Can you work these out from the model? Positions are in its coordinate system, mm. Face numbers are marked on the shaded views. A direction names the side the tool comes from. Round coordinates to 2 decimals unless told otherwise and drop trailing zeros. Write each loop counter-clockwise with the first axis right and the second up, starting at its lowest first coordinate (ties: lowest second). Pieces come first, ordered by that corner, then holes. Notation, with made-up numbers: M 14,-3 L 45,-3 A21 cw 45,13 Z; hole C 10.25,-27.5 d3. An arc over 180 degrees is marked long. Answer in a Markdown table with one row per item. Add a question column.
(1) Suppose I cut it at D-D, the plane z = 15. Write out the boundary of the cut face in (x, y).
(2) Suppose I cut it at A-A, the plane y = 0. Write out the boundary of the cut face in (x, z), then the cut area to 3 significant figures.
(3) Suppose I cut it at C-C, the plane z = 5. Write out the boundary of the cut face in (x, y), then the cut area to 3 significant figures.
(4) For the marked faces 1, 2 and 3, which set-ups out of +Z, -Z, +X, -X, +Y, -Y let a thin tool reach every point of the face, with its end or its side?
(5) If I drill on probe 1 along Y at (x, z) = (0, 7); probe 2 along Z at (x, y) = (-38.5, -17), over which ranges is the centre line in solid material (lowest first)?
(6) I'm going to push flat-ended pins straight in: pin 1 (12 mm diameter, centred on x = 8.5, z = 4.5, fed in from -Y); pin 2 (1.5 mm diameter, centred on x = -15, z = 14.5, fed in from -Y); pin 3 (12 mm diameter, centred on y = -33, z = -15.5, fed in from -X); pin 4 (12 mm diameter, centred on x = 6.5, y = 40, fed in from +Z). Where does each tip first touch, or does it pass through?
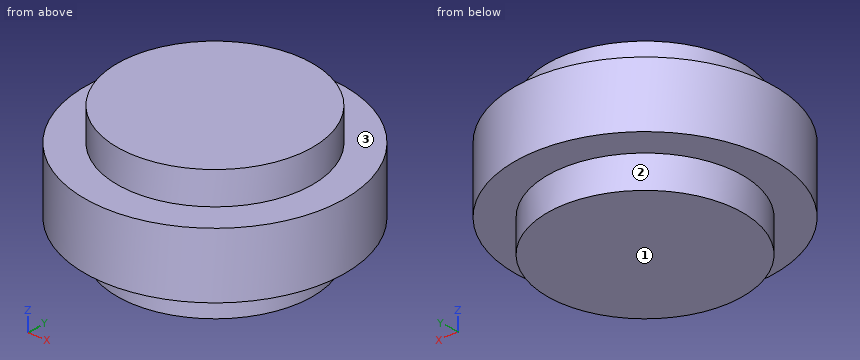
from build123d import *

# Parameters (mm, degrees)
F0_R     = 38.1
F1_DEPTH = 25.4
F0_R_2   = 50.8
F2_DEPTH = 12.7


with BuildPart() as f1:
    # F0 (on Top) → F1 (new body, symmetric)
    with BuildSketch(Plane.XY):
        Circle(F0_R)
    extrude(amount=F1_DEPTH, both=True)

    # F0 (on Top) → F2 (join, symmetric)
    with BuildSketch(Plane.XY):
        Circle(F0_R_2)
        Circle(F0_R, mode=Mode.SUBTRACT)
    extrude(amount=F2_DEPTH, both=True)


solid = f1.part
Calculated:
| question | item | result |
|---|---|---|
| 1 | outline | C 0,0 d76.2 |
| 2 | outline | M -50.8,-12.7 L -38.1,-12.7 L -38.1,-25.4 L 38.1,-25.4 L 38.1,-12.7 L 50.8,-12.7 L 50.8,12.7 L 38.1,12.7 L 38.1,25.4 L -38.1,25.4 L -38.1,12.7 L -50.8,12.7 Z |
| 2 | area | 4,520 mm² |
| 3 | outline | C 0,0 d101.6 |
| 3 | area | 8,110 mm² |
| 4 | face 1 | -Z, +X, -X, +Y, -Y |
| 4 | face 2 | -Z |
| 4 | face 3 | +Z |
| 5 | probe 1 | -50.8 to 50.8 |
| 5 | probe 2 | -12.7 to 12.7 |
| 6 | pin 1 | y = -50.74 |
| 6 | pin 2 | y = -35.33 |
| 6 | pin 3 | x = -42.59 |
| 6 | pin 4 | z = 25.4 |
